```python
from build123d import *

# Parameters (mm, degrees)
SKETCH1_W           = 18
SKETCH1_H           = 32.75
SKETCH1_W_2         = 23
SKETCH1_H_2         = 15.25
SKETCH1_H_3         = 47.05
BOSS_EXTRUDE1_DEPTH = 40
CUT_EXTRUDE1_REACH  = 106.244
SKETCH2_R           = 2.75
CUT_EXTRUDE2_REACH  = 94.276
SKETCH3_W           = 9
SKETCH3_H           = 15.25
SKETCH4_W           = 10
SKETCH4_H           = 15.25
CUT_EXTRUDE3_DEPTH  = 102.645904984
CUT_EXTRUDE4_REACH  = 106.244
SKETCH6_R           = 3.25
CHAMFER1_SIZE       = 1
CUT_EXTRUDE5_REACH  = 106.244
SKETCH7_R           = 3.3
SKETCH8_R           = 2.75
CUT_EXTRUDE6_DEPTH  = 101.542975886
SKETCH9_W           = 23
SKETCH9_H           = 25
SKETCH9_W_2         = 18
SKETCH9_H_2         = 10.7
BOSS_EXTRUDE2_DEPTH = 5


with BuildPart() as part:
    # Sketch1 → Boss-Extrude1 (new body)
    with BuildSketch(Plane.XY):
        Polygon((0, 0), (0, 64), (23, 64), (23, 78.3), (56, 78.3), (56, 0), align=None)
        with Locations((14, 21.375)):
            Rectangle(SKETCH1_W, SKETCH1_H, mode=Mode.SUBTRACT)
        with Locations((39.5, 64.675)):
            Rectangle(SKETCH1_W_2, SKETCH1_H_2, mode=Mode.SUBTRACT)
        with Locations((14, 50.375)):
            Rectangle(SKETCH1_W, SKETCH1_H_2, mode=Mode.SUBTRACT)
        with Locations((39.5, 28.525)):
            Rectangle(SKETCH1_W_2, SKETCH1_H_3, mode=Mode.SUBTRACT)
    extrude(amount=BOSS_EXTRUDE1_DEPTH)

    # Cut-Extrude1: up to this face of the body (flat: up to its plane)
    cut_extrude1_end = Plane(part.part.faces().sort_by_distance((14, 37.75, 20))[0])
    # Sketch2 → Cut-Extrude1 (cut, up to the picked face)
    with BuildSketch(Plane(origin=(0, 78.3, 0), x_dir=(1, 0, 0), z_dir=(0, 1, 0)), mode=Mode.PRIVATE) as cut_extrude1_sk1:
        with Locations(Location((14, -15, 0), (0, 0, 180))):
            Circle(SKETCH2_R)
    cut_extrude1_tool1 = split(extrude(cut_extrude1_sk1.sketch, amount=-CUT_EXTRUDE1_REACH, mode=Mode.PRIVATE), bisect_by=cut_extrude1_end, keep=Keep.BOTH, mode=Mode.PRIVATE)
    # Sketch2 → Cut-Extrude1 (cut, up to the picked face)
    with BuildSketch(Plane(origin=(0, 78.3, 0), x_dir=(1, 0, 0), z_dir=(0, 1, 0)), mode=Mode.PRIVATE) as cut_extrude1_sk2:
        with Locations(Location((37, -30, 0), (0, 0, 180))):
            Circle(SKETCH2_R)
    cut_extrude1_tool2 = split(extrude(cut_extrude1_sk2.sketch, amount=-CUT_EXTRUDE1_REACH, mode=Mode.PRIVATE), bisect_by=cut_extrude1_end, keep=Keep.BOTH, mode=Mode.PRIVATE)
    add(cut_extrude1_tool1.solids().sort_by(Axis((14, 78.3, 15), (0, -1, 0)))[0], mode=Mode.SUBTRACT)
    add(cut_extrude1_tool2.solids().sort_by(Axis((37, 78.3, 30), (0, -1, 0)))[0], mode=Mode.SUBTRACT)

    # Sketch3 → Cut-Extrude2 (cut, up to next)
    with BuildSketch(Plane(origin=(28, 0, 0), x_dir=(0, 0, -1), z_dir=(1, 0, 0)), mode=Mode.PRIVATE) as cut_extrude2_sk1:
        with Locations((-25.5, 64.675)):
            Rectangle(SKETCH3_W, SKETCH3_H)
    cut_extrude2_tool1 = extrude(cut_extrude2_sk1.sketch, amount=-CUT_EXTRUDE2_REACH, mode=Mode.PRIVATE) & part.part
    add(cut_extrude2_tool1.solids().sort_by_distance((28, 64.675, 25.5))[0], mode=Mode.SUBTRACT)

    # Sketch4 → Cut-Extrude3 (cut, through all)
    with BuildSketch(Plane(origin=(5, 0, 0), x_dir=(0, 0, -1), z_dir=(1, 0, 0))):
        with Locations((-10, 50.375)):
            Rectangle(SKETCH4_W, SKETCH4_H)
    extrude(amount=-CUT_EXTRUDE3_DEPTH, mode=Mode.SUBTRACT)

    # Sketch6 → Cut-Extrude4 (cut, up to next)
    with BuildSketch(Plane(origin=(0, 78.3, 0), x_dir=(1, 0, 0), z_dir=(0, 1, 0)), mode=Mode.PRIVATE) as cut_extrude4_sk1:
        with Locations(Location((14, -15, 0), (0, 0, 270))):
            Circle(SKETCH6_R)
    cut_extrude4_tool1 = extrude(cut_extrude4_sk1.sketch, amount=-CUT_EXTRUDE4_REACH, mode=Mode.PRIVATE) & part.part
    # Sketch6 → Cut-Extrude4 (cut, up to next)
    with BuildSketch(Plane(origin=(0, 78.3, 0), x_dir=(1, 0, 0), z_dir=(0, 1, 0)), mode=Mode.PRIVATE) as cut_extrude4_sk2:
        with Locations(Location((37, -30, 0), (0, 0, 270))):
            Circle(SKETCH6_R)
    cut_extrude4_tool2 = extrude(cut_extrude4_sk2.sketch, amount=-CUT_EXTRUDE4_REACH, mode=Mode.PRIVATE) & part.part
    add(cut_extrude4_tool1.solids().sort_by_distance((14, 78.3, 15))[0], mode=Mode.SUBTRACT)
    add(cut_extrude4_tool2.solids().sort_by_distance((37, 78.3, 30))[0], mode=Mode.SUBTRACT)

    # Chamfer1
    chamfer1_edges = [part.edges().sort_by_distance(p)[0] for p in [
        (14, 64, 11.75),
        (37, 78.3, 26.75),
    ]]
    chamfer(chamfer1_edges, length=CHAMFER1_SIZE)

    # Sketch7 → Cut-Extrude5 (cut, up to next)
    with BuildSketch(Plane.XZ, mode=Mode.PRIVATE) as cut_extrude5_sk1:
        with Locations((14, 15)):
            Circle(SKETCH7_R)
    cut_extrude5_tool1 = extrude(cut_extrude5_sk1.sketch, amount=-CUT_EXTRUDE5_REACH, mode=Mode.PRIVATE) & part.part
    # Sketch7 → Cut-Extrude5 (cut, up to next)
    with BuildSketch(Plane.XZ, mode=Mode.PRIVATE) as cut_extrude5_sk2:
        with Locations((44, 15)):
            Circle(SKETCH7_R)
    cut_extrude5_tool2 = extrude(cut_extrude5_sk2.sketch, amount=-CUT_EXTRUDE5_REACH, mode=Mode.PRIVATE) & part.part
    # Sketch7 → Cut-Extrude5 (cut, up to next)
    with BuildSketch(Plane.XZ, mode=Mode.PRIVATE) as cut_extrude5_sk3:
        with BuildLine():
            Line((11.25, 35), (11.25, 40))
            Line((11.25, 40), (16.75, 40))
            Line((16.75, 40), (16.75, 35))
            ThreePointArc((16.75, 35), (14, 32.25), (11.25, 35))
        make_face()
    cut_extrude5_tool3 = extrude(cut_extrude5_sk3.sketch, amount=-CUT_EXTRUDE5_REACH, mode=Mode.PRIVATE) & part.part
    # Sketch7 → Cut-Extrude5 (cut, up to next)
    with BuildSketch(Plane.XZ, mode=Mode.PRIVATE) as cut_extrude5_sk4:
        with BuildLine():
            Line((41.25, 35), (41.25, 40))
            Line((41.25, 40), (46.75, 40))
            Line((46.75, 40), (46.75, 35))
            ThreePointArc((46.75, 35), (44, 32.25), (41.25, 35))
        make_face()
    cut_extrude5_tool4 = extrude(cut_extrude5_sk4.sketch, amount=-CUT_EXTRUDE5_REACH, mode=Mode.PRIVATE) & part.part
    add(cut_extrude5_tool1.solids().sort_by_distance((14, 0, 15))[0], mode=Mode.SUBTRACT)
    add(cut_extrude5_tool2.solids().sort_by_distance((44, 0, 15))[0], mode=Mode.SUBTRACT)
    add(cut_extrude5_tool3.solids().sort_by_distance((14, 0, 36.393769))[0], mode=Mode.SUBTRACT)
    add(cut_extrude5_tool4.solids().sort_by_distance((44, 0, 36.393769))[0], mode=Mode.SUBTRACT)

    # Sketch8 → Cut-Extrude6 (cut, through all)
    with BuildSketch(Plane(origin=(0, 5, 0), x_dir=(1, 0, 0), z_dir=(0, 1, 0))):
        with Locations(Location((37, -30, 0), (0, 0, 180))):
            Circle(SKETCH8_R)
    extrude(amount=-CUT_EXTRUDE6_DEPTH, mode=Mode.SUBTRACT)

    # Sketch9 → Boss-Extrude2 (add)
    with BuildSketch(Plane(origin=(0, 0, 0), x_dir=(-1, 0, 0), z_dir=(0, 0, -1))):
        Polygon((-23, 78.3), (0, 64), (-23, 64), align=None)
        with Locations((-39.5, 39.55)):
            Rectangle(SKETCH9_W, SKETCH9_H)
        with Locations((-14, 32.4)):
            Rectangle(SKETCH9_W_2, SKETCH9_H_2)
    extrude(amount=-BOSS_EXTRUDE2_DEPTH)


solid = part.part
```
Here's how the part is built. I have some questions about the finished solid (model axes, mm). A direction names the side the tool comes from. Coordinates: 2 decimals unless noted, no trailing zeros. Loops run counter-clockwise (first coordinate to the right, second up) from the corner with the lowest first, then second, coordinate; pieces in that order, holes last. Notation, with made-up numbers: M -33,10.5 L 21,10.5 A15 cw 21,15.5 Z; hole C 8,76 d2. An arc over 180 degrees is marked long. One line per item, written item: value.
1. Imagine slicing it at D-D (z = 38.5). State how many separate pieces and enclosed holes the cut face has, and give its area (3 significant figures).
Geometry says:
separate pieces: 1
enclosed holes: 2
area: 1,700 mm2
2. Please list where these lines run through material, in increasing order: probe 1 along Y at (x, z) = (5.5, 8); probe 2 along Y at (x, z) = (30, 28); probe 3 along X at (y, z) = (6, 38.5).
Geometry says:
probe 1: y = 0 to 5, 37.75 to 42.75, 58 to 64
probe 2: y = 0 to 5, 52.05 to 57.05, 72.3 to 78.3
probe 3: x = 0 to 5, 23 to 28, 51 to 56
3. Imagine slicing it at A-A (y = 55). List the corners of the cut face in (x, z) for me, and give its area (3 significant figures).
Geometry says:
outline: M 0,0 L 5,0 L 5,5 L 0,5 Z; M 0,15 L 5,15 L 5,40 L 0,40 Z; M 23,0 L 56,0 L 56,40 L 23,40 Z; hole C 37,30 d5.5
area: 1,450 mm2
4. Imagine slicing it at B-B (x = 37). List the corners of the cut face in (y, z) for me.
Geometry says:
outline: M 0,0 L 5,0 L 5,27.25 L 0,27.25 Z; M 0,32.75 L 5,32.75 L 5,40 L 0,40 Z; M 27.05,0 L 57.05,0 L 57.05,27.25 L 52.05,27.25 L 52.05,5 L 27.05,5 Z; M 52.05,32.75 L 57.05,32.75 L 57.05,40 L 52.05,40 Z; M 72.3,0 L 78.3,0 L 78.3,25.75 L 77.3,26.75 L 72.3,26.75 Z; M 72.3,33.25 L 77.3,33.25 L 78.3,34.25 L 78.3,40 L 72.3,40 Z
5. Imagine slicing it at C-C (y = 23.5). List the corners of the cut face in (x, z) for me, and give its area (3 significant figures).
Geometry says:
outline: M 0,0 L 5,0 L 5,40 L 0,40 Z; M 23,0 L 28,0 L 28,40 L 23,40 Z; M 51,0 L 56,0 L 56,40 L 51,40 Z
area: 600 mm2
6. On a 3-axis mill with a long thin cutter (end or side, diameter ignored), from which of +Z, -Z, +X, -X, +Y, -Y can I reach the whole of each face in a straight line? I mean faces 1 (the cylindrical face through (44.06, 2.46, 32.25)), 2 (the flat face through (28, 65, 35)), 3 (the flat face through (3, 57.05, 26)), 4 (the flat face through (11, 64, 35)). Say none if no direction works.
Geometry says:
face 1: +Z, -Y
face 2: +Z, -Z
face 3: -X, +Y
face 4: +Z, -X, +Y
7. Will these pins go through, and if not, where does the flat tip stop? pin 1 Ø7 at (x, z) = (15.5, 19.5) entering from +Y; pin 2 Ø7.5 at (x, z) = (14, 15) entering from +Y.
Geometry says:
pin 1: stops at y = 64
pin 2: stops at y = 63.5
8. Thinking about a two-plate mould opening in X: for faces 5 (the flat face through (28, 0, 20)), 6 (the flat face through (11.66, 71.25, 2.46)), 7 (the flat face through (51, 28, 20)), 8 (the flat face through (56, 40, 20)), which applies, +X half, -X half, draft (parallel to the pull), parting line (faces both ways), or undercut?
Geometry says:
face 5: draft
face 6: -X half
face 7: undercut
face 8: +X half
